from build123d import *

# Parameters (mm, degrees)
REVOLVE_4_ANGLE          = 60
PATTERN_CIRCULAR_1_COUNT = 4


with BuildPart() as part:
    # 草图1 → 旋转2 (revolve)
    with BuildSketch(Plane.XY, mode=Mode.PRIVATE) as revolve_2_sk:
        with BuildLine():
            Line((-4.981080731, -19.736358929), (-8.981080731, -19.736358929))
            Line((-8.981080731, -19.736358929), (-8.981080731, -21.736358929))
            Line((-8.981080731, -21.736358929), (-10.981080731, -21.736358929))
            Line((-10.981080731, -21.736358929), (-10.981080731, -19.736358929))
            Line((-10.981080731, -19.736358929), (-11.981080731, -19.736358929))
            add(Edge.make_bspline(
                [(-11.981080731, -19.736358929), (-14.105079515, -29.836776521), (-22.689787766, -34.041464812)],
                knots=[0, 0, 0, 1, 1, 1], degree=2))
            Line((-22.689787766, -34.041464812), (-26.167714154, -31.046896542))
            ThreePointArc((-26.167714154, -31.046896542), (-27.689787766, -30.481913457), (-29.211861379, -31.046896542))
            Line((-29.211861379, -31.046896542), (-32.689787766, -34.041464812))
            Line((-32.689787766, -34.041464812), (-36.167714154, -31.046896542))
            ThreePointArc((-36.167714154, -31.046896542), (-37.689787766, -30.481913457), (-39.211861379, -31.046896542))
            Line((-39.211861379, -31.046896542), (-46.981080731, -37.736358929))
            Line((-46.981080731, -37.736358929), (-42.689787766, -37.736358929))
            Line((-42.689787766, -37.736358929), (-37.689787766, -33.431253046))
            Line((-37.689787766, -33.431253046), (-32.689787766, -37.736358929))
            Line((-32.689787766, -37.736358929), (-27.689787766, -33.431253046))
            Line((-27.689787766, -33.431253046), (-22.689787766, -37.736358929))
            add(Edge.make_bspline(
                [(-11.981080731, -23.536358929), (-13.218077622, -28.193488855), (-13.94983801, -29.242750421), (-17.443623259, -35.173249874), (-19.934832658, -36.815558997), (-22.689787766, -37.736358929)],
                knots=[0, 0, 0, 0, 0.485973614, 0.585973614, 1, 1, 1, 1], degree=3))
            Line((-11.981080731, -23.536358929), (-9.781080731, -27.736358929))
            Line((-9.781080731, -27.736358929), (-4.981080731, -27.736358929))
            Line((-4.981080731, -27.736358929), (-4.981080731, -19.736358929))
        make_face()
    revolve(revolve_2_sk.sketch.rotate(Axis((7.759097512, -12.736358929, 0), (-1, 0, 0)), 180), axis=Axis((7.759097512, -12.736358929, 0), (-1, 0, 0)))


with BuildPart() as body_2:
    # 草图3 → 旋转4 (revolve)
    with BuildSketch(Plane(origin=(0, -12.639611974, 1.105822759), x_dir=(1, 0, 0), z_dir=(0, -0.9961946980917459, 0.08715574274765504))):
        with BuildLine():
            Line((-11.981080731, -8.768373779), (-11.981080731, -7.110046822))
            Line((-11.981080731, -7.110046822), (-18.981080731, -7.110046822))
            Line((-18.981080731, -7.110046822), (-18.981080731, -21.291174479))
            add(Edge.make_bspline(
                [(-11.981080731, -8.768373779), (-12.626813815, -12.193567325), (-14.690315158, -16.799816788), (-17.609024266, -20.330987822), (-18.981080731, -21.291174479)],
                knots=[0, 0, 0, 0, 0.528344687, 0.796807345, 0.796807345, 0.796807345, 0.796807345], degree=3))
        make_face()
    revolve(axis=Axis((-4.981080731, -12.736358929, 0), (-1, 0, 0)), revolution_arc=REVOLVE_4_ANGLE)


with BuildPart() as pattern_circular_1_1:
    # 阵列(圆周)1: pattern copy
    add(body_2.part.rotate(Axis((-56.121874835, -12.736358929, 0), (1, 0, 0)), 1 * 360 / PATTERN_CIRCULAR_1_COUNT))


with BuildPart() as pattern_circular_1_2:
    # 阵列(圆周)1: pattern copy
    add(body_2.part.rotate(Axis((-56.121874835, -12.736358929, 0), (1, 0, 0)), 2 * 360 / PATTERN_CIRCULAR_1_COUNT))


with BuildPart() as pattern_circular_1_3:
    # 阵列(圆周)1: pattern copy
    add(body_2.part.rotate(Axis((-56.121874835, -12.736358929, 0), (1, 0, 0)), 3 * 360 / PATTERN_CIRCULAR_1_COUNT))


with BuildPart() as part_1:
    add(part.part)

    # Combine 1: union 阵列(圆周)1_1, body 2, 阵列(圆周)1_2, 阵列(圆周)1_3
    add(pattern_circular_1_1.part)
    add(body_2.part)
    add(pattern_circular_1_2.part)
    add(pattern_circular_1_3.part)

    # 草图5 → 旋转5 (revolve)
    with BuildSketch(Plane(origin=(0, -12.639611974, 1.105822759), x_dir=(1, 0, 0), z_dir=(0, -0.9961946980917459, 0.08715574274765475))):
        with BuildLine():
            Line((-14.981080731, 4.889953178), (-17.481080731, 4.889953178))
            add(Edge.make_bspline(
                [(-14.981080731, 4.889953178), (-16.231080731, 4.089953178), (-17.481080731, 4.889953178)],
                knots=[0, 0, 0, 1, 1, 1], degree=2))
        make_face()
    revolve(axis=Axis((-56.121874835, -12.736358929, 0), (1, 0, 0)))


solid = part_1.part
Could you check a few things on this model? Use its own coordinates, in mm. A direction names the side the tool comes from. Give positions to 0.01 mm unless a question says otherwise; leave off trailing zeros. Loops run counter-clockwise (first coordinate to the right, second up) from the corner with the lowest first, then second, coordinate; pieces in that order, holes last. Notation, with made-up numbers: M -21,-4.75 L -15,-4.75 A30 cw -15,21.25 Z; hole C -34,76 d8. An arc over 180 degrees is marked long. Answer as a JSON object with one key per item and string values.
Q1. For P1, Ø13, axis at y = -20.5, z = -12, coming from the -X side; P2, Ø8.5, axis at y = -12.74, z = 0, coming from the -X side; P3, Ø1.3, axis at y = -10, z = 5.5, coming from the +X side; P4, Ø8, axis at y = -25, z = 5, coming from the -X side, each with a flat end and sliding along its axis, tell me the tip position at first contact or that it passes through.
Values found:
{"P1": "stops at x = -42.09", "P2": "passes through", "P3": "stops at x = -11.98", "P4": "stops at x = -18.98"}
Q2. If I drill on probe 1 along X at (y, z) = (4, -12); probe 2 along X at (y, z) = (4, -10); probe 3 along Z at (x, y) = (-20.5, 3), over which ranges is the centre line in solid material (lowest first)? Write a range as [from, to].
Values found:
{"probe 1": "x = [-41.86, -33.52], [-31.86, -23.52], [-21.36, -16.42]", "probe 2": "x = [-40.59, -34.79], [-30.59, -24.79], [-19.66, -15.71]", "probe 3": "z = [-18.25, -12.46], [12.46, 18.25]"}
Q3. For faces 3 (the cylindrical face through (-18.242, -17.676, 3.405)), 4 (the cylindrical face through (-13.502, -17.676, 3.405)), 5 (the conical face through (-36, -27.38, 11.23)), 6 (the cylindrical face through (-16.25, -18.65, -1.02)), which set-ups out of +Z, -Z, +X, -X, +Y, -Y let a thin tool reach every point of the face, with its end or its side?
Values found:
{"face 3": "-X", "face 4": "+X", "face 5": "none", "face 6": "+X, -X"}
Q4. Suppose I cut it at A-A, the plane x = -8. List the corners of the cut face in (y, z) for me, plus the area to 3 significant figures.
Values found:
{"outline": "C -12.74,0 d30; hole C -12.74,0 d14", "area": "553 mm²"}
Q5. Suppose I cut it at B-B, the plane x = -40.5. List the corners of the cut face in (y, z) for me, plus the area to 3 significant figures.
Values found:
{"outline": "C -12.74,0 d46.23; hole C -12.74,0 d38.84", "area": "494 mm²"}
Q6. If we mould it in two halves opening along Y, with no side actions, what happens to faces 1 (the conical face through (-27.933, -29.325, 12.72)), 2 (the flat face through (-11.981, -9, 5))? For each: pulls with the +Y half, pulls with the -Y half, needs draft (parallel to the pull), parting line crosses it, or undercut.
Values found:
{"face 1": "parting line crosses it", "face 2": "undercut"}
